```python
from build123d import *

# Parameters (mm, degrees)
SKETCH1_R                         = 12.5
SKETCH1_R_2                       = 11.5
BOSS_EXTRUDE1_DEPTH               = 14
BOSS_EXTRUDE2_START               = 1
SKETCH2_R                         = 12.5
SKETCH2_R_2                       = 7.5
BOSS_EXTRUDE2_DEPTH               = 1
F_80_0_0135_DIAMETER_HOLE1_REACH  = 31.497
F_80_0_0135_DIAMETER_HOLE1_BORE_R = 0.17145
F_80_0_0135_DIAMETER_HOLE2_REACH  = 31.833
F_80_0_0135_DIAMETER_HOLE2_BORE_R = 0.17145


with BuildPart() as part:
    # Sketch1 → Boss-Extrude1 (new body)
    with BuildSketch(Plane(origin=(0, 0, 0), x_dir=(1, 0, 0), z_dir=(0, 1, 0))):
        with Locations(Location((0, 0, 0), (0, 0, 270))):
            Circle(SKETCH1_R)
        with Locations(Location((0, 0, 0), (0, 0, 270))):
            Circle(SKETCH1_R_2, mode=Mode.SUBTRACT)
    extrude(amount=BOSS_EXTRUDE1_DEPTH)

    # Sketch2 → Boss-Extrude2 (add)
    with BuildSketch(Plane(origin=(0, 0, 0), x_dir=(-1, 0, 0), z_dir=(0, -1, 0)).offset(BOSS_EXTRUDE2_START)):
        with Locations(Location((0, 0, 0), (0, 0, 90))):
            Circle(SKETCH2_R)
        with Locations(Location((0, 0, 0), (0, 0, 90))):
            Circle(SKETCH2_R_2, mode=Mode.SUBTRACT)
    extrude(amount=-BOSS_EXTRUDE2_DEPTH)

    # #80 (0.0135) Diameter Hole1 bore (on position points) → #80 (0.0135) Diameter Hole1 (cut, up to next)
    with BuildSketch(Plane(origin=(12.499604816, 8.291561976, 0.099395334), x_dir=(-0.00795162675, 0, 0.999968385316), z_dir=(0.999968385316, 0, 0.00795162675)), mode=Mode.PRIVATE) as f_80_0_0135_diameter_hole1_sk1:
        Circle(F_80_0_0135_DIAMETER_HOLE1_BORE_R)
    f_80_0_0135_diameter_hole1_tool1 = extrude(f_80_0_0135_diameter_hole1_sk1.sketch, amount=-F_80_0_0135_DIAMETER_HOLE1_REACH, mode=Mode.PRIVATE) & part.part
    add(f_80_0_0135_diameter_hole1_tool1.solids().sort_by_distance((12.499605, 8.291562, 0.099395))[0], mode=Mode.SUBTRACT)

    # #80 (0.0135) Diameter Hole2 bore (on position points) → #80 (0.0135) Diameter Hole2 (cut, up to next)
    with BuildSketch(Plane(origin=(12.5, 3.570714214, 0), x_dir=(0, 0, 1), z_dir=(1, 0, 0)), mode=Mode.PRIVATE) as f_80_0_0135_diameter_hole2_sk1:
        Circle(F_80_0_0135_DIAMETER_HOLE2_BORE_R)
    f_80_0_0135_diameter_hole2_tool1 = extrude(f_80_0_0135_diameter_hole2_sk1.sketch, amount=-F_80_0_0135_DIAMETER_HOLE2_REACH, mode=Mode.PRIVATE) & part.part
    add(f_80_0_0135_diameter_hole2_tool1.solids().sort_by_distance((12.5, 3.570714, 0))[0], mode=Mode.SUBTRACT)


solid = part.part
```
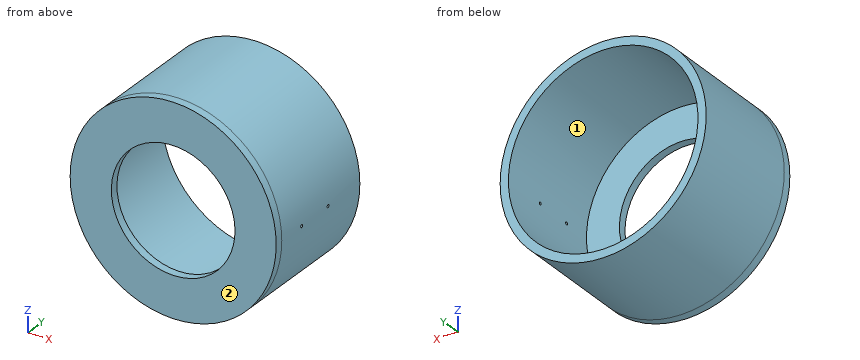
Check sheet for the modelled part. Datum: model origin and axes. Units: mm. Face numbers are marked on the shaded views. Round coordinates to 2 decimals unless told otherwise and drop trailing zeros. Write each loop counter-clockwise with the first axis right and the second up, starting at its lowest first coordinate (ties: lowest second). Pieces come first, ordered by that corner, then holes. Notation, with made-up numbers: (49.25, -21.75) -> (69.25, -21.75) arc R19 ccw to (69.25, 10.25) -> close; hole circle Ø1 at (88.25, 66.25). An arc over 180 degrees is marked (long way). Put each result on its own line as item: value.
(1) Sectioned sample at B-B (z = 2.25). Enter the section's corners in (x, y).
Values found:
outline: (-12.3, -1) -> (-7.15, -1) -> (-7.15, 0) -> (-11.28, 0) -> (-11.28, 14) -> (-12.3, 14) -> close; (7.15, -1) -> (12.3, -1) -> (12.3, 14) -> (11.28, 14) -> (11.28, 0) -> (7.15, 0) -> close
(2) Sectioned sample at C-C (y = 1.75). Enter the section's corners in (x, z), plus the area to 3 significant figures.
Values found:
outline: circle Ø25 at (0, 0); hole circle Ø23 at (0, 0)
area: 75.4 mm^2
(3) Sectioned sample at D-D (x = -8.5). Enter the section's corners in (y, z).
Values found:
outline: (-1, -9.17) -> (14, -9.17) -> (14, -7.75) -> (0, -7.75) -> (0, 7.75) -> (14, 7.75) -> (14, 9.17) -> (-1, 9.17) -> close
(4) Sectioned sample at A-A (x = 0). Enter the section's corners in (y, z).
Values found:
outline: (-1, -12.5) -> (14, -12.5) -> (14, -11.5) -> (0, -11.5) -> (0, -7.5) -> (-1, -7.5) -> close; (-1, 7.5) -> (0, 7.5) -> (0, 11.5) -> (14, 11.5) -> (14, 12.5) -> (-1, 12.5) -> close
(5) Go/stop test with flat-tipped pins: pin 1 Ø1.5 at (x, y) = (-4, 9.5) entering from -Z; pin 2 Ø1.5 at (x, z) = (-7.5, 3) entering from +Y; pin 3 Ø2 at (x, y) = (-6, 5) entering from +Z. Record where each tip stops, or that it passes through.
Values found:
pin 1: stops at z = -12.07
pin 2: stops at y = 0
pin 3: stops at z = 11.46
(6) Material ranges on line 1 (X direction, y = 10, z = 0); line 2 (Y direction, x = 12, z = 0); line 3 (Y direction, x = -6.5, z = -7.5), recorded low to high.
Values found:
line 1: x = -12.5 to -11.5, 11.5 to 12.5
line 2: y = -1 to 3.4, 3.74 to 8.15, 8.43 to 14
line 3: y = -1 to 0
(7) Mould release check, pull along X, two halves, no side actions. Record for the marked faces 1 and 2: released by +X, released by -X, zero draft, split by the parting line, or undercut.
Values found:
face 1: undercut
face 2: zero draft
